The listing builds one solid part. Answer for the finished solid, in the listing's coordinates (mm). Face numbers are marked on the shaded views. Give positions to 0.01 mm unless a question says otherwise; leave off trailing zeros. Loops run counter-clockwise (first coordinate to the right, second up) from the corner with the lowest first, then second, coordinate; pieces in that order, holes last. Notation, with made-up numbers: (39, -10.5) - (85, -10.5) arc R15 ccw to (85, 5.5) - close; hole circle Ø2 at (20.25, -9.5). An arc over 180 degrees is marked (long way). Write item = value, one per line. Start each with the question number.
1) The part is cut by section D-D on x = 4.5. Write down the section's boundary in (y, z).
2) The mould has two halves that part along Y. Classify the marked faces 1, 2, 3 and 4: +Y half, -Y half, draft (parallel to the pull), parting line (faces both ways), or undercut.
3) A flat-ended cylindrical pin translates along its axis: P1, Ø5, axis at x = -3, y = 2, coming from the -Z side. Find the tip coordinate at first contact, or state that the pin passes through.
4) The part is cut by section B-B on x = 0. Write down the section's boundary in (y, z).
5) The part is cut by section C-C on z = 1.75. Write down the section's boundary in (x, y), plus the area to 4 significant figures.
6) Consider probe 1 along Y at (x, z) = (0, 1.45); probe 2 along X at (y, z) = (-2.5, 0.5); probe 3 along X at (y, z) = (0.5, 0.5). Determine where each line is inside the solid, lowest interval first.
7) The part is cut by section A-A on y = 0. Write down the section's boundary in (x, z).
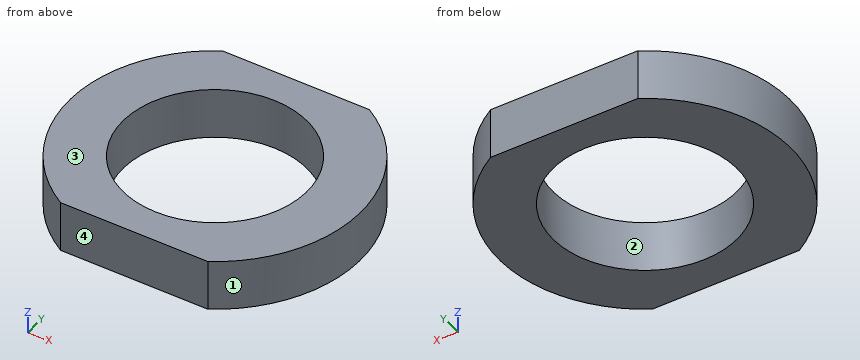
from build123d import *

# Parameters (mm, degrees)
CIRCLE_R         = 3.6
EXTRUDE004_DEPTH = 2
CIRCLE002_R      = 3.5
EXTRUDE002_DEPTH = 2
CIRCLE003_R      = 5.7
EXTRUDE003_DEPTH = 2
RECTANGLE_W      = 25.8
RECTANGLE_H      = 9.8
EXTRUDE_DEPTH    = 2


with BuildPart() as extrude004:
    # Circle → Extrude004 (new body)
    with BuildSketch(Plane.XY.offset(2)):
        Circle(CIRCLE_R)
    extrude(amount=-EXTRUDE004_DEPTH)


with BuildPart() as extrude002:
    # Circle002 (on Rectangle) → Extrude002 (new body)
    with BuildSketch(Plane(origin=(26.064868, 8.047387, 0), x_dir=(1, 0, 0), z_dir=(0, 0, -1))):
        Circle(CIRCLE002_R)
    extrude(amount=-EXTRUDE002_DEPTH)


with BuildPart() as cut001:
    # Circle003 → Extrude003 (new body)
    with BuildSketch(Plane(origin=(26.064868, 8.047387, 0), x_dir=(1, 0, 0), z_dir=(0, 0, -1))):
        Circle(CIRCLE003_R)
    extrude(amount=-EXTRUDE003_DEPTH)

    # Cut001: cut Extrude002
    add(extrude002.part, mode=Mode.SUBTRACT)


with BuildPart() as cut001_1:
    # Cut001 placement: moved
    add(cut001.part.moved(Location((-26.064868, -8.047387, 0))))


with BuildPart() as cut:
    # Rectangle → Extrude (new body)
    with BuildSketch(Plane(origin=(-12.9, 4.9, 0), x_dir=(1, 0, 0), z_dir=(0, 0, -1))):
        with Locations((12.9, 4.9)):
            Rectangle(RECTANGLE_W, RECTANGLE_H)
    extrude(amount=-EXTRUDE_DEPTH)

    # Common: intersect Cut001
    add(cut001_1.part, mode=Mode.INTERSECT)

    # Cut: cut Extrude004
    add(extrude004.part, mode=Mode.SUBTRACT)


solid = cut.part
Answer below:
q1.outline = (-3.5, 0) - (3.5, 0) - (3.5, 2) - (-3.5, 2) - close
q2.face_1 = parting line
q2.face_2 = undercut
q2.face_3 = draft
q2.face_4 = -Y half
q3.P1 = 0
q4.outline = (-4.9, 0) - (-3.6, 0) - (-3.6, 2) - (-4.9, 2) - close; (3.6, 0) - (4.9, 0) - (4.9, 2) - (3.6, 2) - close
q5.outline = (-2.91, -4.9) - (2.91, -4.9) arc R5.7 ccw to (2.91, 4.9) - (-2.91, 4.9) arc R5.7 ccw to start; hole circle Ø7.2 at (0, 0)
q5.area = 55.05 mm2
q6.probe_1 = -4.9 to -3.6, 3.6 to 4.9
q6.probe_2 = -5.12 to -2.59, 2.59 to 5.12
q6.probe_3 = -5.68 to -3.57, 3.57 to 5.68
q7.outline = (-5.7, 0) - (-3.6, 0) - (-3.6, 2) - (-5.7, 2) - close; (3.6, 0) - (5.7, 0) - (5.7, 2) - (3.6, 2) - close
